Model file for the job. Use its own axes, mm. A direction names the side the tool comes from. Round coordinates to 2 decimals unless told otherwise and drop trailing zeros. Write each loop counter-clockwise with the first axis right and the second up, starting at its lowest first coordinate (ties: lowest second). Pieces come first, ordered by that corner, then holes.
```python
from build123d import *

# Parameters (mm, degrees)
SKETCH1_W               = 44
SKETCH1_H               = 6
BOSS_EXTRUDE1_DEPTH     = 277
SKETCH4_W               = 9
SKETCH4_H               = 6
BOSS_EXTRUDE2_DEPTH     = 6
SKETCH5_W               = 9
SKETCH5_H               = 6
BOSS_EXTRUDE3_DEPTH     = 6
SKETCH6_W               = 9.5
SKETCH6_H               = 6
BOSS_EXTRUDE4_DEPTH     = 6
SKETCH7_R               = 1.6
CUT_EXTRUDE1_DEPTH      = 286.346184868
SKETCH8_R               = 2.5
CUT_EXTRUDE2_DEPTH      = 12
SKETCH9_R               = 1.6
CUT_EXTRUDE3_DEPTH      = 12
CUT_EXTRUDE4_DEPTH      = 286.346184868
CUT_EXTRUDE4_DEPTH_BACK = 286.346184868
SKETCH11_R              = 2.75
SKETCH7_2_R             = 1.6
BOSS_EXTRUDE5_DEPTH     = 6
BOSS_EXTRUDE5_2_DEPTH   = 6
SKETCH12_R              = 1.25
SKETCH12_R_2            = 10
CUT_EXTRUDE5_DEPTH      = 286.346184868


with BuildPart() as part:
    # Sketch1 → Boss-Extrude1 (new body)
    with BuildSketch(Plane.XY):
        with Locations((-8.02006689, 7.52173913)):
            Rectangle(SKETCH1_W, SKETCH1_H)
    extrude(amount=BOSS_EXTRUDE1_DEPTH)

    # Sketch4 → Boss-Extrude2 (add)
    with BuildSketch(Plane(origin=(13.97993311, 0, 0), x_dir=(0, 0, -1), z_dir=(1, 0, 0))):
        with Locations((-272, 7.52173913)):
            Rectangle(SKETCH4_W, SKETCH4_H)
        with Locations((-252, 7.52173913)):
            Rectangle(SKETCH4_W, SKETCH4_H)
        with Locations((-232, 7.52173913)):
            Rectangle(SKETCH4_W, SKETCH4_H)
        with Locations((-212, 7.52173913)):
            Rectangle(SKETCH4_W, SKETCH4_H)
        with Locations((-192, 7.52173913)):
            Rectangle(SKETCH4_W, SKETCH4_H)
        with Locations((-172, 7.52173913)):
            Rectangle(SKETCH4_W, SKETCH4_H)
        with Locations((-152, 7.52173913)):
            Rectangle(SKETCH4_W, SKETCH4_H)
        with Locations((-132, 7.52173913)):
            Rectangle(SKETCH4_W, SKETCH4_H)
        with Locations((-112, 7.52173913)):
            Rectangle(SKETCH4_W, SKETCH4_H)
        with Locations((-92, 7.52173913)):
            Rectangle(SKETCH4_W, SKETCH4_H)
        with Locations((-72, 7.52173913)):
            Rectangle(SKETCH4_W, SKETCH4_H)
        with Locations((-52, 7.52173913)):
            Rectangle(SKETCH4_W, SKETCH4_H)
        with Locations((-32, 7.52173913)):
            Rectangle(SKETCH4_W, SKETCH4_H)
        with Locations((-12, 7.52173913)):
            Rectangle(SKETCH4_W, SKETCH4_H)
    extrude(amount=BOSS_EXTRUDE2_DEPTH)

    # Sketch5 → Boss-Extrude3 (add)
    with BuildSketch(Plane.ZY.offset(30.02006689)):
        with Locations((272, 7.52173913)):
            Rectangle(SKETCH5_W, SKETCH5_H)
        with Locations((252, 7.52173913)):
            Rectangle(SKETCH5_W, SKETCH5_H)
        with Locations((232, 7.52173913)):
            Rectangle(SKETCH5_W, SKETCH5_H)
        with Locations((212, 7.52173913)):
            Rectangle(SKETCH5_W, SKETCH5_H)
        with Locations((192, 7.52173913)):
            Rectangle(SKETCH5_W, SKETCH5_H)
        with Locations((172, 7.52173913)):
            Rectangle(SKETCH5_W, SKETCH5_H)
        with Locations((152, 7.52173913)):
            Rectangle(SKETCH5_W, SKETCH5_H)
        with Locations((132, 7.52173913)):
            Rectangle(SKETCH5_W, SKETCH5_H)
        with Locations((112, 7.52173913)):
            Rectangle(SKETCH5_W, SKETCH5_H)
        with Locations((92, 7.52173913)):
            Rectangle(SKETCH5_W, SKETCH5_H)
        with Locations((72, 7.52173913)):
            Rectangle(SKETCH5_W, SKETCH5_H)
        with Locations((52, 7.52173913)):
            Rectangle(SKETCH5_W, SKETCH5_H)
        with Locations((32, 7.52173913)):
            Rectangle(SKETCH5_W, SKETCH5_H)
        with Locations((12, 7.52173913)):
            Rectangle(SKETCH5_W, SKETCH5_H)
    extrude(amount=BOSS_EXTRUDE3_DEPTH)

    # Sketch6 → Boss-Extrude4 (add)
    with BuildSketch(Plane.XY.offset(277)):
        with Locations((-18.02006689, 7.52173913)):
            Rectangle(SKETCH6_W, SKETCH6_H)
        with Locations((1.97993311, 7.52173913)):
            Rectangle(SKETCH6_W, SKETCH6_H)
    extrude(amount=BOSS_EXTRUDE4_DEPTH)

    # Sketch7 → Cut-Extrude1 (cut, through all)
    with BuildSketch(Plane.XZ.offset(-4.52173913)):
        with Locations(Location((16.97993311, 252, 0), (0, 0, 270))):
            Circle(SKETCH7_R)
        with Locations(Location((-33.02006689, 252, 0), (0, 0, 90))):
            Circle(SKETCH7_R)
        with Locations(Location((-33.02006689, 212, 0), (0, 0, 90))):
            Circle(SKETCH7_R)
        with Locations(Location((16.97993311, 212, 0), (0, 0, 270))):
            Circle(SKETCH7_R)
        with Locations(Location((-33.02006689, 172, 0), (0, 0, 90))):
            Circle(SKETCH7_R)
        with Locations(Location((16.97993311, 172, 0), (0, 0, 270))):
            Circle(SKETCH7_R)
        with Locations(Location((-33.02006689, 132, 0), (0, 0, 90))):
            Circle(SKETCH7_R)
        with Locations(Location((16.97993311, 132, 0), (0, 0, 270))):
            Circle(SKETCH7_R)
        with Locations(Location((-33.02006689, 92, 0), (0, 0, 90))):
            Circle(SKETCH7_R)
        with Locations(Location((16.97993311, 92, 0), (0, 0, 270))):
            Circle(SKETCH7_R)
        with Locations(Location((-33.02006689, 52, 0), (0, 0, 90))):
            Circle(SKETCH7_R)
        with Locations(Location((16.97993311, 52, 0), (0, 0, 270))):
            Circle(SKETCH7_R)
        with Locations(Location((-33.02006689, 12, 0), (0, 0, 90))):
            Circle(SKETCH7_R)
        with Locations(Location((16.97993311, 12, 0), (0, 0, 270))):
            Circle(SKETCH7_R)
    extrude(amount=-CUT_EXTRUDE1_DEPTH, mode=Mode.SUBTRACT)

    # Sketch8 → Cut-Extrude2 (cut)
    with BuildSketch(Plane.XZ.offset(-4.52173913)):
        with Locations(Location((-19.02006689, 39, 0), (0, 0, 270))):
            Circle(SKETCH8_R)
        with Locations(Location((2.97993311, 39, 0), (0, 0, 270))):
            Circle(SKETCH8_R)
    extrude(amount=-CUT_EXTRUDE2_DEPTH, mode=Mode.SUBTRACT)

    # Sketch9 → Cut-Extrude3 (cut)
    with BuildSketch(Plane(origin=(0, 4.52173913, 0), x_dir=(-1, 0, 0), z_dir=(0, -1, 0))):
        with Locations(Location((18.02006689, -280, 0), (0, 0, 90))):
            Circle(SKETCH9_R)
        with Locations(Location((-1.97993311, -280, 0), (0, 0, 90))):
            Circle(SKETCH9_R)
    extrude(amount=-CUT_EXTRUDE3_DEPTH, mode=Mode.SUBTRACT)

    # Sketch11 → Cut-Extrude4 (cut, two sides: drawn at the far end of the back side and taken through both)
    with BuildSketch(Plane.XZ.offset(-4.52173913).offset(-CUT_EXTRUDE4_DEPTH_BACK)):
        with Locations(Location((-24.019868524, 226.88732643, 0), (0, 0, 270))):
            Circle(SKETCH11_R)
        with Locations(Location((7.97993311, 227, 0), (0, 0, 270))):
            Circle(SKETCH11_R)
        with Locations(Location((7.97993311, 267, 0), (0, 0, 270))):
            Circle(SKETCH11_R)
        with Locations(Location((-24.02006689, 267, 0), (0, 0, 270))):
            Circle(SKETCH11_R)
    extrude(amount=CUT_EXTRUDE4_DEPTH + CUT_EXTRUDE4_DEPTH_BACK, mode=Mode.SUBTRACT)


with BuildPart() as body_2:
    # Sketch7<2> → Boss-Extrude5 (new, through all)
    with BuildSketch(Plane.XZ.offset(-4.52173913)):
        with Locations(Location((16.97993311, 252, 0), (0, 0, 270))):
            Circle(SKETCH7_2_R)
    extrude(amount=-BOSS_EXTRUDE5_DEPTH)


with BuildPart() as body_3:
    # Sketch7<2> → Boss-Extrude5 2 (new, through all)
    with BuildSketch(Plane.XZ.offset(-4.52173913)):
        with Locations(Location((-33.02006689, 252, 0), (0, 0, 90))):
            Circle(SKETCH7_2_R)
    extrude(amount=-BOSS_EXTRUDE5_2_DEPTH)


with BuildPart() as part_1:
    add(part.part)

    # Combine1: union body 3, body 2
    add(body_3.part)
    add(body_2.part)

    # Sketch12 → Cut-Extrude5 (cut, through all)
    with BuildSketch(Plane(origin=(0, 10.52173913, 0), x_dir=(1, 0, 0), z_dir=(0, 1, 0))):
        with Locations(Location((4.97993311, -159.533243973, 0), (0, 0, 270))):
            Circle(SKETCH12_R)
        with Locations(Location((-21.02006689, -159.533243973, 0), (0, 0, 270))):
            Circle(SKETCH12_R)
        with Locations(Location((-21.02006689, -93.533243973, 0), (0, 0, 270))):
            Circle(SKETCH12_R)
        with Locations(Location((4.97993311, -93.533243973, 0), (0, 0, 270))):
            Circle(SKETCH12_R)
        with Locations(Location((-8.02006689, -170.956644726, 0), (0, 0, 270))):
            Circle(SKETCH12_R_2)
    extrude(amount=-CUT_EXTRUDE5_DEPTH, mode=Mode.SUBTRACT)


solid = part_1.part
```
1) Cut at A-A on z = 125. List the corners of the cut face in (x, y).
2) Flat gauge pins, fed straight in: pin 1 Ø1.8 at (y, z) = (6.5, 204.5) entering from -X; pin 2 Ø3 at (x, y) = (-34.5, 8.5) entering from +Z; pin 3 Ø4 at (x, z) = (-21.02, 93.53) entering from -Y; pin 4 Ø2 at (x, z) = (4.98, 93.53) entering from -Y. Where does each tip first touch, or does it go through?
3) Which spindle directions (+Z, -Z, +X, -X, +Y, -Y) get a long thin tool onto all of the face, cutting with end or side? Do faces 1 (the face through (-33, 7, 16.5)), 2 (the face through (-36.02, 8, 112)), 3 (the face through (13.98, 7, 182)). Say none if no direction does.
4) Pull direction Z, two halves, no side cores. Call faces 4 (the face through (-30.02, 7, 102)), 5 (the face through (-36.02, 8, 172)): released by +Z, released by -Z, zero draft, split by the parting line, or undercut.
5) Cut at B-B on y = 8.25. Give the number of separate pieces and of enclosed holes in the cut face, and give its area (3 significant figures).
6) Wall check: probe 1 along X at (y, z) = (5.75, 92); probe 2 along Z at (x, y) = (-23.5, 6); probe 3 along Z at (x, y) = (-24, 5.75). Give the ranges that are in metal, low to high.
Result sheet:
1. outline: (-30.02, 4.52) - (13.98, 4.52) - (13.98, 10.52) - (-30.02, 10.52) - close
2. pin 1: stops at x = -30.02
2. pin 2: stops at z = 276.5
2. pin 3: stops at y = 4.52
2. pin 4: passes through
3. face 1: -X, +Y, -Y
3. face 2: +Z, -Z, -X, +Y, -Y
3. face 3: +X, +Y, -Y
4. face 4: undercut
4. face 5: zero draft
5. separate pieces: 1
5. enclosed holes: 25
5. area: 13,200 mm2
6. probe 1: x = -36.02 to -34.62, -31.42 to 15.38, 18.58 to 19.98
6. probe 2: z = 0 to 224.19, 229.59 to 264.3, 269.7 to 277
6. probe 3: z = 0 to 224.14, 229.64 to 264.25, 269.75 to 277
